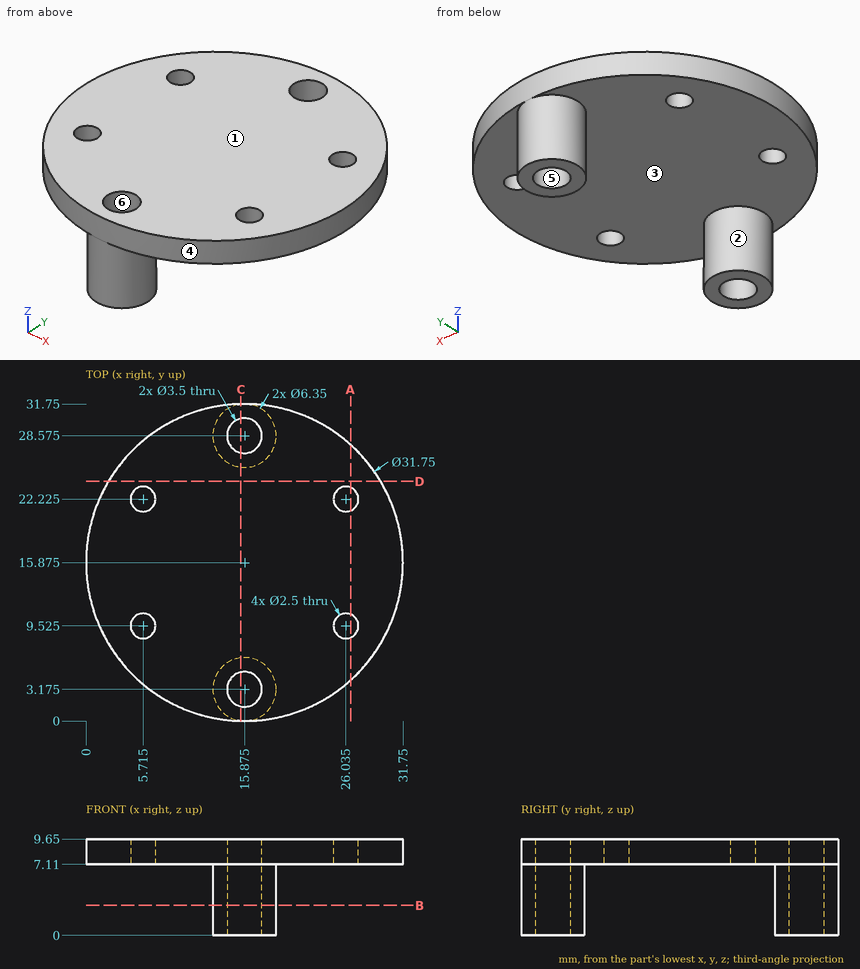
The drawing under review shows one solid part. Ordinate dimensions are in mm from its lowest x, y, z. A direction names the side the tool comes from. Coordinates: 2 decimals unless noted, no trailing zeros. Loops run counter-clockwise (first coordinate to the right, second up) from the corner with the lowest first, then second, coordinate; pieces in that order, holes last. Notation, with made-up numbers: (12.5, 3) - (56.5, 3) arc R16 ccw to (56.5, 10) - close; hole circle Ø3 at (82.25, -8). An arc over 180 degrees is marked (long way). Return JSON: item names as keys, results as strings.
Item 1: Take a section at D-D (y = 24). Give the boundary of the cut face in (x, z), then the cut area to 3 significant figures.
Determined:
{"outline": "(2.24, 7.11) - (29.51, 7.11) - (29.51, 9.65) - (2.24, 9.65) - close", "area": "69.3 mm2"}
Item 2: Take a section at A-A (x = 26.5). Give the boundary of the cut face in (y, z).
Determined:
{"outline": "(4.08, 7.11) - (8.36, 7.11) - (8.36, 9.65) - (4.08, 9.65) - close; (10.69, 7.11) - (21.06, 7.11) - (21.06, 9.65) - (10.69, 9.65) - close; (23.39, 7.11) - (27.67, 7.11) - (27.67, 9.65) - (23.39, 9.65) - close"}
Item 3: Take a section at B-B (z = 3). Give the boundary of the cut face in (x, y) (3 decimals), then the cut area to 3 significant figures.
Determined:
{"outline": "circle Ø6.35 at (15.875, 3.175); circle Ø6.35 at (15.875, 28.575); hole circle Ø3.5 at (15.875, 3.175); hole circle Ø3.5 at (15.875, 28.575)", "area": "44.1 mm2"}
Item 4: Mouldability with a two-part tool opening along X and no side actions: class the marked faces 3, 4, 5 and 6 as pulls with the +X half, pulls with the -X half, needs draft (parallel to the pull), parting line crosses it, or undercut.
Determined:
{"face 3": "needs draft", "face 4": "parting line crosses it", "face 5": "undercut", "face 6": "undercut"}
Item 5: Take a section at C-C (x = 15.5). State how many separate pieces and enclosed holes the cut face has, then the cut area to 3 significant figures.
Determined:
{"separate pieces": "3", "enclosed holes": "0", "area": "104 mm2"}
Item 6: Insertion check: pin 1 (5 mm diameter, centred on y = 4, z = 8, fed in from -X). The pin has a flat end and moves straight along its axis. Give the tip position at first contact, or say it passes through.
Determined:
{"pin 1": "stops at x = 3.06"}
Item 7: For line 1 (X direction, y = 23, z = 9); line 2 (Z direction, x = 26, y = 5.5); line 3 (X direction, y = 27.5, z = 3), list the stretches that pass through material, from the lowest coordinate up.
Determined:
{"line 1": "x = 1.69 to 4.73, 6.7 to 25.05, 27.02 to 30.06", "line 2": "z = 7.11 to 9.65", "line 3": "x = 12.89 to 14.49, 17.26 to 18.86"}
Item 8: For the marked faces 1 and 2, list the 3-axis set-ups (+Z, -Z, +X, -X, +Y, -Y) from which the entire face can be reached by the end or side of a thin tool; tool diameter is ignored.
Determined:
{"face 1": "+Z, +X, -X, +Y, -Y", "face 2": "-Z"}
